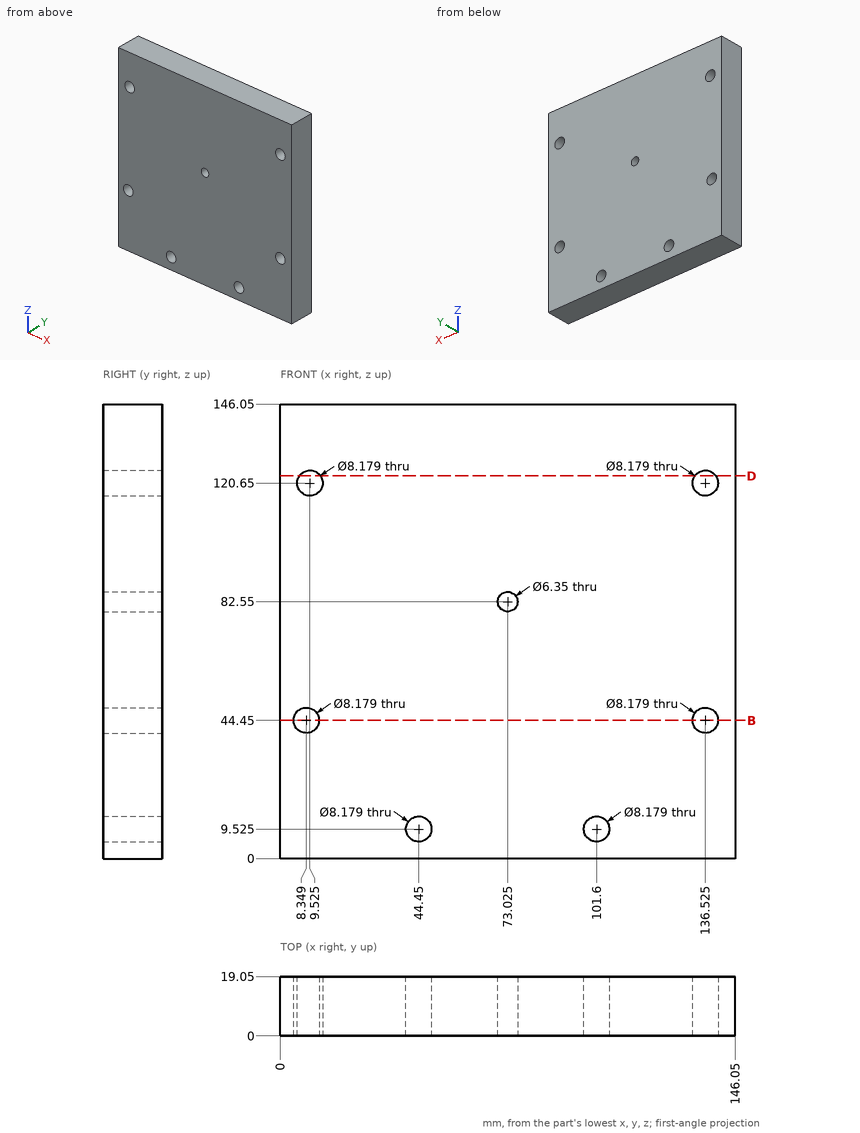
Source: three-view drawing plus pictorial views. Frame: mm from the lowest corner of the part. Round coordinates to 2 decimals unless told otherwise and drop trailing zeros. Order: outer loops, then holes, each group sorted by start corner. A loop starts at its lowest first (then second) coordinate and runs counter-clockwise, first axis right, second up. Notation, with made-up numbers: (-26, 60) - (-1, 60) arc R14 cw to (-1, 65) - close; hole circle Ø1 at (33.5, 38.5). An arc over 180 degrees is marked (long way). Answer in a Markdown table with one row per item.
Item 1: Section query B-B (z = 44.45). Give the number of separate pieces and of enclosed holes in the cut face, then the cut area to 3 significant figures.
Model answer:
| item | result |
|---|---|
| separate pieces | 3 |
| enclosed holes | 0 |
| area | 2,470 mm² |
Item 2: Line query: line 1 (X direction, y = 9.75, z = 44.5); line 2 (Z direction, x = 137, y = 8.5); line 3 (X direction, y = 8, z = 43.5). Output: solid intervals per line, ascending.
Model answer:
| item | result |
|---|---|
| line 1 | x = 0 to 4.26, 12.44 to 132.44, 140.61 to 146.05 |
| line 2 | z = 0 to 40.39, 48.51 to 116.59, 124.71 to 146.05 |
| line 3 | x = 0 to 4.37, 12.33 to 132.55, 140.5 to 146.05 |
Item 3: Section query D-D (z = 123). Return the cut outline in (x, y).
Model answer:
| item | result |
|---|---|
| outline | (0, 0) - (6.18, 0) - (6.18, 19.05) - (0, 19.05) - close; (12.87, 0) - (133.18, 0) - (133.18, 19.05) - (12.87, 19.05) - close; (139.87, 0) - (146.05, 0) - (146.05, 19.05) - (139.87, 19.05) - close |
